Job drawing, mm, ordinate dimensions from the low corner. One solid piece. A direction names the side the tool comes from. Give positions to 0.01 mm unless a question says otherwise; leave off trailing zeros. Write each loop counter-clockwise with the first axis right and the second up, starting at its lowest first coordinate (ties: lowest second). Pieces come first, ordered by that corner, then holes. Notation, with made-up numbers: (48.25, 18.5) -> (88.25, 18.5) arc R28 ccw to (88.25, 44.5) -> close; hole circle Ø6 at (69, 25.25). An arc over 180 degrees is marked (long way). Put each result on its own line as item: value. Start each with the question number.
Item 1: Tool access for the marked faces 1 and 2: list every direction of +Z, -Z, +X, -X, +Y, -Y with a clear straight run to the whole face (end or side of a thin tool).
Item 2: Slice it at A-A, the plane y = 6. List the corners of the cut face in (x, z) (1 decimal).
Item 3: Drill centre lines: line 1 along X through (y, z) = (5.75, 2.75); line 2 along Z through (x, y) = (8.75, 6.5) (1 decimal); line 3 along Y through (x, z) = (14.75, 1.75). Where is each one in solid material? Low to high.
Item 4: Slice it at B-B, the plane x = 8.75. List the corners of the cut face in (y, z) (1 decimal), plus the area to 3 significant figures.
Item 5: Slice it at C-C, the plane x = 3.75. List the corners of the cut face in (y, z) (1 decimal), plus the area to 3 significant figures.
Item 6: Flat gauge pins, fed straight in: pin 1 Ø4 at (x, y) = (7.5, 6) entering from -Z (1 decimal); pin 2 Ø1.6 at (x, z) = (11, 1) entering from +Y; pin 3 Ø0.5 at (y, z) = (0, 0) entering from +X. Where does each tip first touch, or does it go through?
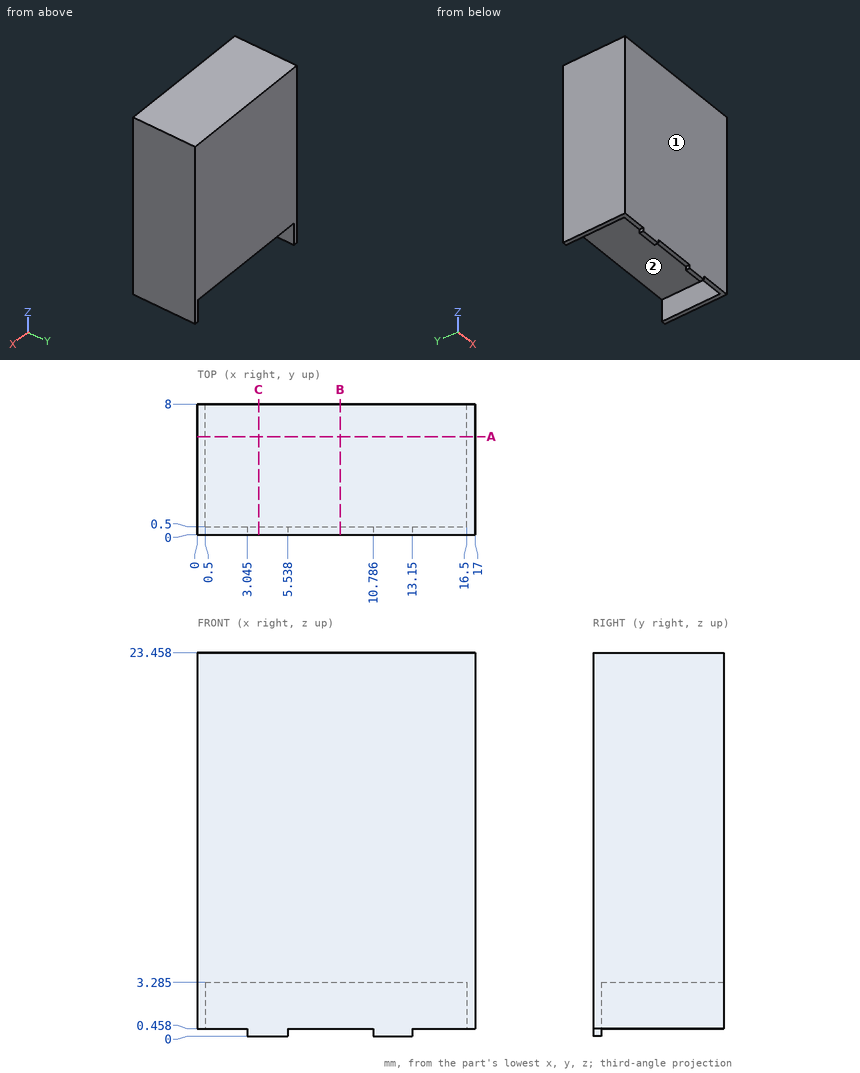
Values follow:
1. face 1: +Z, -Z, +X, -X, -Y
1. face 2: -Z, +Y
2. outline: (0, 0.5) -> (0.5, 0.5) -> (0.5, 3.3) -> (16.5, 3.3) -> (16.5, 0.5) -> (17, 0.5) -> (17, 23.5) -> (0, 23.5) -> close
3. line 1: 0 to 0.5, 16.5 to 17
3. line 2: 3.3 to 23.5
3. line 3: 0 to 0.5
4. outline: (0, 0.5) -> (0.5, 0.5) -> (0.5, 3.3) -> (8, 3.3) -> (8, 23.5) -> (0, 23.5) -> close
4. area: 163 mm2
5. outline: (0, 0) -> (0.5, 0) -> (0.5, 3.3) -> (8, 3.3) -> (8, 23.5) -> (0, 23.5) -> close
5. area: 163 mm2
6. pin 1: z = 3.3
6. pin 2: y = 0.5
6. pin 3: x = 13.15
